Check sheet for the modelled part. Datum: model origin and axes. Units: mm. Coordinates: 2 decimals unless noted, no trailing zeros. Order: outer loops, then holes, each group sorted by start corner. A loop starts at its lowest first (then second) coordinate and runs counter-clockwise, first axis right, second up.
1. Gauge pin test, flat ends, axial feed: pin 1 Ø0.9 at (x, z) = (-3, 1) entering from +Y; pin 2 Ø0.9 at (x, z) = (-75.5, 1) entering from -Y; pin 3 Ø0.9 at (x, z) = (-2.5, 1.5) entering from -Y. Record the tip position at first contact, or that the pin passes through.
2. Cross-section at B-B (x = -52). Enter the section's corners in (y, z).
3. Thickness scan on line 1 (Y direction, x = 28.5, z = 2.3); line 2 (X direction, y = 56.5, z = 1.65). Record the ranges inside material, lowest first.
4. Cross-section at A-A (y = 41). Enter the section's corners in (x, z).
```python
from build123d import *

# Parameters (mm, degrees)
SKETCH_W        = 155
SKETCH_H        = 127
PAD_DEPTH       = 3
SKETCH001_W     = 3
SKETCH001_H     = 10
POCKET_DEPTH    = 403.815171
SKETCH002_W     = 20
SKETCH002_H     = 3
POCKET001_DEPTH = 403.815171


with BuildPart() as part:
    # Sketch → Pad (new body)
    with BuildSketch(Plane.XY):
        Rectangle(SKETCH_W, SKETCH_H)
    extrude(amount=PAD_DEPTH)

    # Sketch001 (on Face6 of Pad) → Pocket (cut, through all)
    with BuildSketch(Plane.XY.offset(3)):
        with Locations((76, 58.5)):
            Rectangle(SKETCH001_W, SKETCH001_H)
        with Locations((76, 38.5)):
            Rectangle(SKETCH001_W, SKETCH001_H)
        with Locations((76, 18.5)):
            Rectangle(SKETCH001_W, SKETCH001_H)
        with Locations((76, -1.5)):
            Rectangle(SKETCH001_W, SKETCH001_H)
        with Locations((76, -21.5)):
            Rectangle(SKETCH001_W, SKETCH001_H)
        with Locations((76, -41.5)):
            Rectangle(SKETCH001_W, SKETCH001_H)
        with Locations((76, -61.5)):
            Rectangle(SKETCH001_W, SKETCH001_H)
    pocket = extrude(amount=-POCKET_DEPTH, mode=Mode.SUBTRACT)

    # Mirrored: Pocket across Sketch001 V_Axis
    add(pocket.mirror(Plane(origin=(0, 0, 3), x_dir=(0, 0, 1), z_dir=(1, 0, 0))), mode=Mode.SUBTRACT)

    # Sketch002 (on Face4 of Mirrored) → Pocket001 (cut, through all)
    with BuildSketch(Plane.XY.offset(3)):
        with Locations((-44.5, -62)):
            Rectangle(SKETCH002_W, SKETCH002_H)
        with Locations((-4.5, -62)):
            Rectangle(SKETCH002_W, SKETCH002_H)
        with Locations((35.5, -62)):
            Rectangle(SKETCH002_W, SKETCH002_H)
    pocket001 = extrude(amount=-POCKET001_DEPTH, mode=Mode.SUBTRACT)

    # Mirrored001: Pocket001 across Sketch002 H_Axis
    add(pocket001.mirror(Plane(origin=(0, 0, 3), x_dir=(0, 0, 1), z_dir=(0, 1, 0))), mode=Mode.SUBTRACT)


solid = part.part
```
Data:
1. pin 1: stops at y = 60.5
1. pin 2: stops at y = -56.5
1. pin 3: stops at y = -60.5
2. outline: (-60.5, 0) - (60.5, 0) - (60.5, 3) - (-60.5, 3) - close
3. line 1: y = -60.5 to 60.5
3. line 2: x = -74.5 to 74.5
4. outline: (-74.5, 0) - (74.5, 0) - (74.5, 3) - (-74.5, 3) - close
